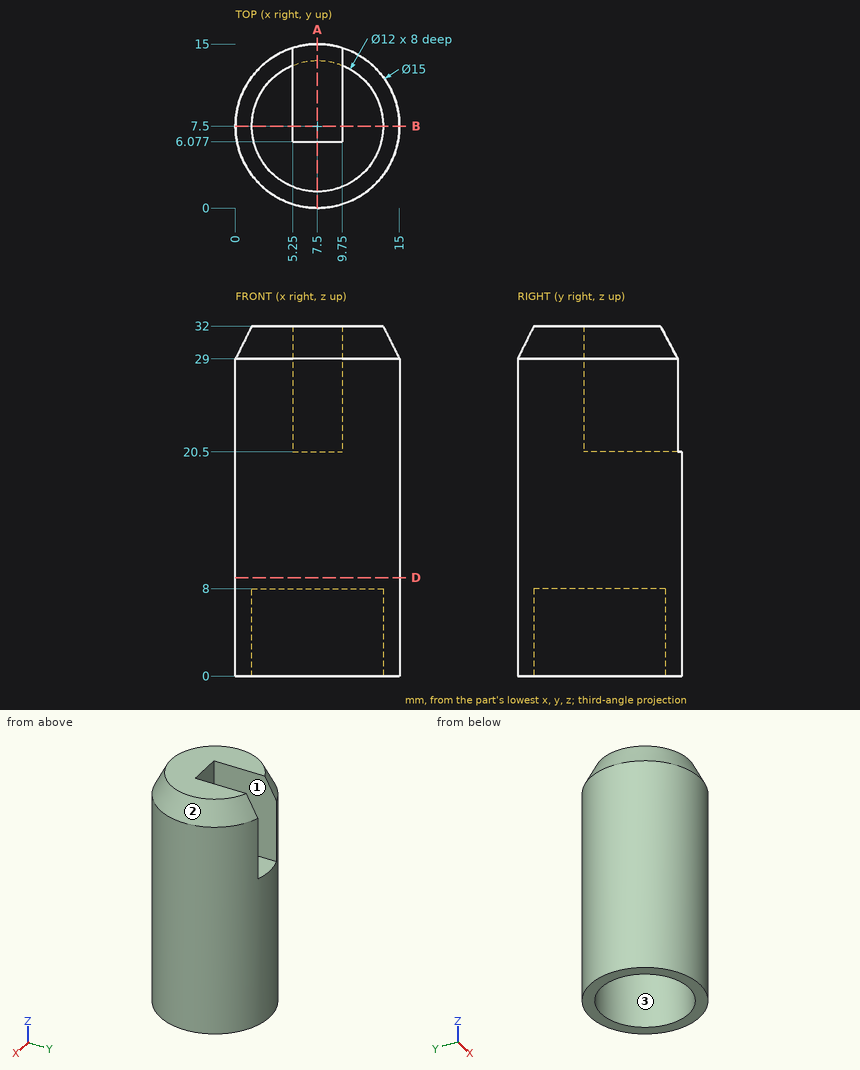
Could you check a few things on this drawing? It's one solid part, dimensions in mm from its lowest x, y, z. Round coordinates to 2 decimals unless told otherwise and drop trailing zeros. Order: outer loops, then holes, each group sorted by start corner. A loop starts at its lowest first (then second) coordinate and runs counter-clockwise, first axis right, second up.
Q1. Thinking about a two-plate mould opening in Y: for the marked faces 1, 2 and 3, which applies, released by +Y, released by -Y, zero draft, split by the parting line, or undercut?
Geometry says:
face 1: zero draft
face 2: split by the parting line
face 3: undercut
Q2. Imagine slicing it at B-B, the plane y = 7.5. List the corners of the cut face in (x, z) for me.
Geometry says:
outline: (0, 0) - (1.5, 0) - (1.5, 8) - (13.5, 8) - (13.5, 0) - (15, 0) - (15, 29) - (13.5, 32) - (9.75, 32) - (9.75, 20.5) - (5.25, 20.5) - (5.25, 32) - (1.5, 32) - (0, 29) - close
Q3. I'm going to push flat-ended pins straight in: P1, Ø6, axis at x = 5, z = 15, coming from the -Y side; P2, Ø1, axis at x = 11, z = 22, coming from the -Y side; P3, Ø1.5, axis at x = 10.5, z = 22.5, coming from the -Y side (1 decimal); P4, Ø4, axis at x = 2.5, z = 14.5, coming from the +Y side. Where does each tip first touch, or does it pass through?
Geometry says:
P1: stops at y = 0
P2: stops at y = 0.63
P3: stops at y = 0.3
P4: stops at y = 14.37
Q4. Imagine slicing it at D-D, the plane z = 9. List the corners of the cut face in (x, y) for me, then the cut area to 3 significant figures.
Geometry says:
outline: circle Ø15 at (7.5, 7.5)
area: 177 mm2
Q5. Imagine slicing it at A-A, the plane x = 7.5. List the corners of the cut face in (y, z) for me.
Geometry says:
outline: (0, 0) - (1.5, 0) - (1.5, 8) - (13.5, 8) - (13.5, 0) - (15, 0) - (15, 20.5) - (6.08, 20.5) - (6.08, 32) - (1.5, 32) - (0, 29) - close
Q6. Please list where these lines run through material, in increasing order: probe 1 along Y at (x, z) = (7.5, 2.5); probe 2 along Z at (x, y) = (2.75, 9.75); probe 3 along X at (y, z) = (5.5, 6.5).
Geometry says:
probe 1: y = 0 to 1.5, 13.5 to 15
probe 2: z = 8 to 32
probe 3: x = 0.27 to 1.84, 13.16 to 14.73
